Read the model definition and answer for the solid it produces. Units are mm, in the model's axes. Face numbers are marked on the shaded views. A direction names the side the tool comes from. Give positions to 0.01 mm unless a question says otherwise; leave off trailing zeros. Loops run counter-clockwise (first coordinate to the right, second up) from the corner with the lowest first, then second, coordinate; pieces in that order, holes last. Notation, with made-up numbers: (-13.5, -4.5) - (10.5, -4.5) arc R28 ccw to (10.5, 32.5) - close; hole circle Ø5 at (-26.75, 3.5). An arc over 180 degrees is marked (long way). Write each question's results on one line, items separated by ' | '. Start each with the question number.
Q1. The part is cut by section B-B, the plane y = 7. Write down the section's boundary in (x, z).
Q2. For the marked faces 4 and 5, determine the directions among +Z, -Z, +X, -X, +Y, -Y from which every point of the face is accessible in a straight line to the end or side of a thin tool.
Q3. The part is cut by section D-D, the plane x = 97.5. Write down the section's boundary in (y, z).
Q4. The part is cut by section A-A, the plane x = 104. Write down the section's boundary in (y, z).
Q5. The part is cut by section C-C, the plane z = -75. Write down the section's boundary in (x, y), plus the area to 3 significant figures.
Q6. Determine the mould class of the marked faces 1, 2 and 3 for opening direction Z: +Z half, -Z half, draft (parallel to the pull), parting line (faces both ways), or undercut.
Q7. Given pin 1 (1 mm diameter, centred on y = 16.5, z = -75.5, fed in from -X); pin 2 (0.8 mm diameter, centred on x = 104.5, y = 16.5, fed in from -Z); pin 3 (1 mm diameter, centred on y = 15.5, z = -48.5, fed in from -X), each flat-ended and moving along its own axis, determine where each tip first touches the part or whether it passes through.
Q8. Find the intervals of material crossed by line 1 (Z direction, x = 106.5, y = 2.75); line 2 (Y direction, x = 111, z = -65.5); line 3 (X direction, y = 11, z = -65.5), in increasing order. Write a range as from..to.
```python
from build123d import *

# Parameters (mm, degrees)
BOSS_EXTRUDE1_DEPTH = 15
BOSS_EXTRUDE2_DEPTH = 2
SKETCH4_W           = 6.62021856
SKETCH4_H           = 1.294383367
CUT_EXTRUDE1_DEPTH  = 1


with BuildPart() as part:
    # Sketch1 → Boss-Extrude1 (new body)
    with BuildSketch(Plane(origin=(0, 0, 0), x_dir=(1, 0, 0), z_dir=(0, 1, 0))):
        with BuildLine():
            Line((95.929523932, 46.874695494), (108.027641063, 46.874695494))
            ThreePointArc((108.027641063, 46.874695494), (113.077675482, 48.185488052), (116.852687564, 51.786919511))
            Line((116.852687564, 51.786919511), (116.852687564, 73.318230601))
            ThreePointArc((116.852687564, 73.318230601), (113.077675482, 76.919662059), (108.027641063, 78.230454618))
            Line((108.027641063, 78.230454618), (95.929523932, 78.230454618))
            ThreePointArc((95.929523932, 78.230454618), (80.25164437, 62.552575056), (95.929523932, 46.874695494))
        make_face()
        with BuildLine():
            Line((95.929523932, 76.230454618), (108.027641063, 76.230454618))
            ThreePointArc((108.027641063, 76.230454618), (111.866170296, 75.300049315), (114.852687564, 72.715349081))
            Line((114.852687564, 72.715349081), (114.852687564, 52.389801031))
            ThreePointArc((114.852687564, 52.389801031), (111.866170296, 49.805100796), (108.027641063, 48.874695494))
            Line((108.027641063, 48.874695494), (95.929523932, 48.874695494))
            ThreePointArc((95.929523932, 48.874695494), (82.25164437, 62.552575056), (95.929523932, 76.230454618))
        make_face(mode=Mode.SUBTRACT)
    extrude(amount=BOSS_EXTRUDE1_DEPTH)

    # Sketch3 → Boss-Extrude2 (add)
    with BuildSketch(Plane(origin=(0, 15, 0), x_dir=(1, 0, 0), z_dir=(0, 1, 0))):
        with BuildLine():
            Line((108.027641063, 76.230454618), (106.652687564, 76.230454618))
            Line((106.652687564, 76.230454618), (106.652687564, 72.730454618))
            Line((106.652687564, 72.730454618), (98.652687564, 72.730454618))
            Line((98.652687564, 72.730454618), (98.652687564, 76.230454618))
            Line((98.652687564, 76.230454618), (95.929523932, 76.230454618))
            ThreePointArc((95.929523932, 76.230454618), (82.25164437, 62.552575056), (95.929523932, 48.874695494))
            Line((95.929523932, 48.874695494), (98.652687564, 48.874695494))
            Line((98.652687564, 48.874695494), (98.652687564, 52.374695494))
            Line((98.652687564, 52.374695494), (106.652687564, 52.374695494))
            Line((106.652687564, 52.374695494), (106.652687564, 48.874695494))
            Line((106.652687564, 48.874695494), (108.027641063, 48.874695494))
            ThreePointArc((108.027641063, 48.874695494), (111.866170296, 49.805100796), (114.852687564, 52.389801031))
            Line((114.852687564, 52.389801031), (114.852687564, 72.715349081))
            ThreePointArc((114.852687564, 72.715349081), (111.866170296, 75.300049315), (108.027641063, 76.230454618))
        make_face()
        with BuildLine():
            Line((98.652687564, 76.230454618), (98.652687564, 78.230454618))
            Line((98.652687564, 78.230454618), (95.929523932, 78.230454618))
            ThreePointArc((95.929523932, 78.230454618), (80.25164437, 62.552575056), (95.929523932, 46.874695494))
            Line((95.929523932, 46.874695494), (98.652687564, 46.874695494))
            Line((98.652687564, 46.874695494), (98.652687564, 48.874695494))
            Line((98.652687564, 48.874695494), (95.929523932, 48.874695494))
            ThreePointArc((95.929523932, 48.874695494), (82.25164437, 62.552575056), (95.929523932, 76.230454618))
            Line((95.929523932, 76.230454618), (98.652687564, 76.230454618))
        make_face()
        with BuildLine():
            Line((108.027641063, 78.230454618), (106.652687564, 78.230454618))
            Line((106.652687564, 78.230454618), (106.652687564, 76.230454618))
            Line((106.652687564, 76.230454618), (108.027641063, 76.230454618))
            ThreePointArc((108.027641063, 76.230454618), (111.866170296, 75.300049315), (114.852687564, 72.715349081))
            Line((114.852687564, 72.715349081), (114.852687564, 52.389801031))
            ThreePointArc((114.852687564, 52.389801031), (111.866170296, 49.805100796), (108.027641063, 48.874695494))
            Line((108.027641063, 48.874695494), (106.652687564, 48.874695494))
            Line((106.652687564, 48.874695494), (106.652687564, 46.874695494))
            Line((106.652687564, 46.874695494), (108.027641063, 46.874695494))
            ThreePointArc((108.027641063, 46.874695494), (113.077675482, 48.185488052), (116.852687564, 51.786919511))
            Line((116.852687564, 51.786919511), (116.852687564, 73.318230601))
            ThreePointArc((116.852687564, 73.318230601), (113.077675482, 76.919662059), (108.027641063, 78.230454618))
        make_face()
    extrude(amount=BOSS_EXTRUDE2_DEPTH)

    # Sketch4 → Cut-Extrude1 (cut)
    with BuildSketch(Plane(origin=(0, 17, 0), x_dir=(1, 0, 0), z_dir=(0, 1, 0))):
        with Locations((102.652687564, 54.099354042)):
            Rectangle(SKETCH4_W, SKETCH4_H)
        Polygon((103.319354231, 68.217634105), (103.319354231, 66.268916157), (101.986020897, 66.268916157), (101.986020897, 68.217634105), (99.934738846, 68.217634105), (99.934738846, 69.550967439), (101.986020897, 69.550967439), (101.986020897, 71.499685387), (103.319354231, 71.499685387), (103.319354231, 69.550967439), (105.370636282, 69.550967439), (105.370636282, 68.217634105), align=None)
    extrude(amount=-CUT_EXTRUDE1_DEPTH, mode=Mode.SUBTRACT)


solid = part.part
```
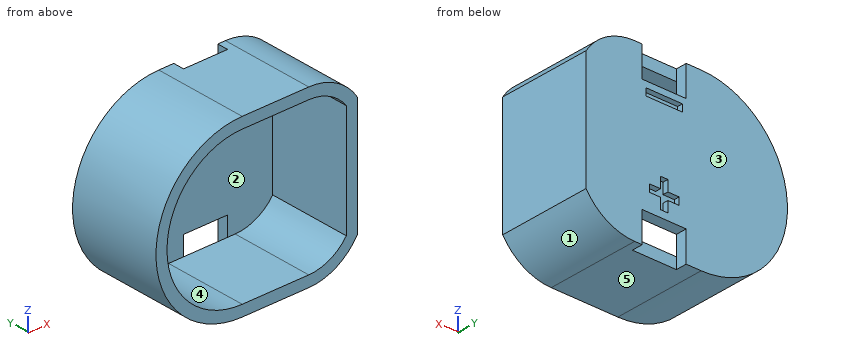
Check sheet entries:
1) outline: (95.93, -78.23) - (108.03, -78.23) arc R10.38 ccw to (116.85, -73.32) - (116.85, -51.79) arc R10.38 ccw to (108.03, -46.87) - (95.93, -46.87) arc R15.68 ccw to start; hole (95.93, -76.23) - (108.03, -76.23) arc R8.38 ccw to (114.85, -72.72) - (114.85, -52.39) arc R8.38 ccw to (108.03, -48.87) - (95.93, -48.87) arc R13.68 ccw to start
2) face 4: -Y | face 5: -Z, +X, -X, +Y, -Y
3) outline: (0, -78.23) - (17, -78.23) - (17, -46.87) - (0, -46.87) - (0, -48.87) - (15, -48.87) - (15, -76.23) - (0, -76.23) - close
4) outline: (0, -78.23) - (15, -78.23) - (15, -76.23) - (0, -76.23) - close; (0, -48.87) - (15, -48.87) - (15, -46.87) - (0, -46.87) - close; (15, -72.73) - (17, -72.73) - (17, -69.55) - (16, -69.55) - (16, -68.22) - (17, -68.22) - (17, -54.75) - (16, -54.75) - (16, -53.45) - (17, -53.45) - (17, -52.37) - (15, -52.37) - close
5) outline: (86.4, 0) - (90.26, 0) - (90.26, 15) - (98.65, 15) - (98.65, 17) - (86.4, 17) - close; (106.65, 15) - (112.4, 15) - (112.4, 0) - (115.55, 0) - (115.55, 17) - (106.65, 17) - close | area: 148 mm^2
6) face 1: -Z half | face 2: undercut | face 3: draft
7) pin 1: stops at x = 86.4 | pin 2: stops at z = -72.73 | pin 3: stops at x = 88.05
8) line 1: z = -78.23..-76.23, -48.87..-46.87 | line 2: y = 15..17 | line 3: x = 80.53..82.57, 114.85..116.85
